Input: part model. Units: mm. Frame: model coordinates. Face numbers are marked on the shaded views. A direction names the side the tool comes from. Coordinates: 2 decimals unless noted, no trailing zeros. Loops run counter-clockwise (first coordinate to the right, second up) from the corner with the lowest first, then second, coordinate; pieces in that order, holes last. Notation, with made-up numbers: (-36.5, 69.5) - (-9.5, 69.5) arc R22 cw to (-9.5, 85.5) - close; hole circle Ø7 at (87, 70). An arc over 180 degrees is marked (long way). Use a Markdown table: item, result. Add a question column.
1. Draft query along X for the marked faces 1, 2 and 3. Return one class per face: released by +X, released by -X, zero draft, split by the parting line, or undercut.
2. Access query for the marked faces 4, 5 and 6. Directions: +Z, -Z, +X, -X, +Y, -Y. A direction counts if a zero-diameter tool reaches every point of the face in a straight line with its end or side. Return the directions, or none.
3. Ray query, L1, parallel to X at y = 1, z = -20; L2, parallel to X at y = 8.5, z = -13 (3 decimals); L3, parallel to Z at x = 38.5, y = -7 (3 decimals). Return the intervals inside material, ascending. Write a range as [from, to].
4. Section query C-C on z = 12. Return the cut outline in (x, y) (3 decimals), then the cut area to 3 significant figures.
5. Section query D-D on x = 21.5. Return the cut outline in (y, z) (3 decimals).
6. Contact query for flat-ended pins moving along their axis: P1, Ø4.5, axis at x = 52.125, z = 20.025, coming from the -Y side; P2, Ø3.5, axis at x = -45.5, z = 19, coming from the +Y side; P3, Ø1.5, axis at x = -12.5, z = -7.5, coming from the -Y side. Output: stop coordinate, or through.
7. Section query A-A on z = -7. Return the cut outline in (x, y) (3 decimals).
8. Section query B-B on y = 12. Return the cut outline in (x, z) (3 decimals), then the cut area to 3 significant figures.
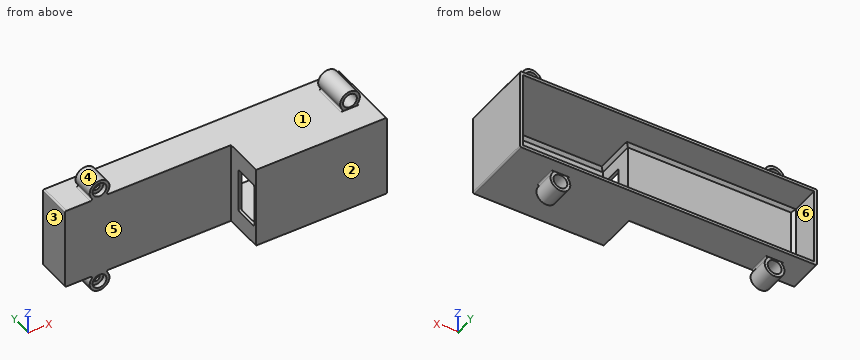
```python
from build123d import *

# Parameters (mm, degrees)
SKETCH1_W                      = 120.25
SKETCH1_H                      = 33.25
BOSS_EXTRUDE1_DEPTH            = 14
CUT_EXTRUDE1_REACH             = 67.133
CUT_EXTRUDE1_START             = 1.2
SKETCH1_3_W                    = 117.85
SKETCH1_3_H                    = 30.85
SKETCH2_W                      = 53
SKETCH2_H                      = 33.25
BOSS_EXTRUDE2_DEPTH            = 16
SKETCH2_3_W                    = 50.6
SKETCH2_3_H                    = 30.85
CUT_EXTRUDE2_DEPTH             = 14.8
CUT_EXTRUDE2_DIRECTION_2_REACH = 66.4
SKETCH3_W                      = 18
SKETCH3_H                      = 10
CUT_EXTRUDE4_DEPTH             = 8.325
SKETCH1_4_R                    = 4
BOSS_EXTRUDE3_DEPTH            = 9
BOSS_EXTRUDE4_START            = -5
SKETCH1_5_R                    = 4
BOSS_EXTRUDE4_DEPTH            = 5
CUT_EXTRUDE5_START             = 9
SKETCH1_6_R                    = 2.8
CUT_EXTRUDE5_DEPTH             = 6
CUT_EXTRUDE6_START             = 2
SKETCH1_7_R                    = 2.8
CUT_EXTRUDE6_DEPTH             = 7
CUT_EXTRUDE7_DEPTH             = 67.694949209
CUT_EXTRUDE7_DEPTH_BACK        = 67.694949209
SKETCH1_8_R                    = 1.3
CUT_EXTRUDE8_START             = 2
SKETCH1_9_R                    = 2.8
CUT_EXTRUDE8_DEPTH             = 2
FILLET1_R                      = 0.6
CHAMFER1_SIZE                  = 1.2


with BuildPart() as part:
    # Sketch1 → Boss-Extrude1 (new body)
    with BuildSketch(Plane(origin=(0, 0, 0), x_dir=(1, 0, 0), z_dir=(0, 1, 0))):
        Rectangle(SKETCH1_W, SKETCH1_H)
    extrude(amount=BOSS_EXTRUDE1_DEPTH)

    # Sketch1<3> → Cut-Extrude1 (cut, up to next)
    with BuildSketch(Plane(origin=(0, 0, 0), x_dir=(1, 0, 0), z_dir=(0, 1, 0)).offset(CUT_EXTRUDE1_START), mode=Mode.PRIVATE) as cut_extrude1_sk1:
        Rectangle(SKETCH1_3_W, SKETCH1_3_H)
    cut_extrude1_tool1 = extrude(cut_extrude1_sk1.sketch, amount=CUT_EXTRUDE1_REACH, mode=Mode.PRIVATE) & part.part
    add(cut_extrude1_tool1.solids().sort_by_distance((0, 1.2, 0))[0], mode=Mode.SUBTRACT)

    # Sketch2 → Boss-Extrude2 (add)
    with BuildSketch(Plane(origin=(0, 0, 0), x_dir=(1, 0, 0), z_dir=(0, 1, 0))):
        with Locations((33.625, 0)):
            Rectangle(SKETCH2_W, SKETCH2_H)
    extrude(amount=-BOSS_EXTRUDE2_DEPTH)

    # Sketch2<3> → Cut-Extrude2 (cut)
    with BuildSketch(Plane(origin=(0, 0, 0), x_dir=(1, 0, 0), z_dir=(0, 1, 0))):
        with Locations((33.625, 0)):
            Rectangle(SKETCH2_3_W, SKETCH2_3_H)
    extrude(amount=-CUT_EXTRUDE2_DEPTH, mode=Mode.SUBTRACT)

    # Sketch2<3> → Cut-Extrude2 direction 2 (cut, up to next)
    with BuildSketch(Plane(origin=(0, 0, 0), x_dir=(1, 0, 0), z_dir=(0, 1, 0)), mode=Mode.PRIVATE) as cut_extrude2_direction_2_sk1:
        with Locations((33.625, 0)):
            Rectangle(SKETCH2_3_W, SKETCH2_3_H)
    cut_extrude2_direction_2_tool1 = extrude(cut_extrude2_direction_2_sk1.sketch, amount=CUT_EXTRUDE2_DIRECTION_2_REACH, mode=Mode.PRIVATE) & part.part
    add(cut_extrude2_direction_2_tool1.solids().sort_by_distance((33.625, 0, 0))[0], mode=Mode.SUBTRACT)

    # Sketch3 → Cut-Extrude4 (cut)
    with BuildSketch(Plane(origin=(0, 0, 0), x_dir=(0, 0, -1), z_dir=(1, 0, 0))):
        with Locations((0, -9.8)):
            Rectangle(SKETCH3_W, SKETCH3_H)
    extrude(amount=CUT_EXTRUDE4_DEPTH, mode=Mode.SUBTRACT)

    # Sketch1<4> → Boss-Extrude3 (add)
    with BuildSketch(Plane(origin=(0, 0, 0), x_dir=(1, 0, 0), z_dir=(0, 1, 0))):
        with Locations((-46.125, -20.025)):
            Circle(SKETCH1_4_R)
        with Locations((52.125, -20.025)):
            Circle(SKETCH1_4_R)
        with Locations((-46.125, 20.025)):
            Circle(SKETCH1_4_R)
        with Locations((40.625, 20.025)):
            Circle(SKETCH1_4_R)
    extrude(amount=BOSS_EXTRUDE3_DEPTH)

    # Sketch1<5> → Boss-Extrude4 (add)
    with BuildSketch(Plane(origin=(0, 0, 0), x_dir=(1, 0, 0), z_dir=(0, 1, 0)).offset(BOSS_EXTRUDE4_START)):
        with Locations((52.125, -20.025)):
            Circle(SKETCH1_5_R)
    extrude(amount=BOSS_EXTRUDE4_DEPTH)

    # Sketch1<6> → Cut-Extrude5 (cut)
    with BuildSketch(Plane(origin=(0, 0, 0), x_dir=(1, 0, 0), z_dir=(0, 1, 0)).offset(CUT_EXTRUDE5_START)):
        with Locations(Location((-46.125, 20.025, 0), (0, 0, 270))):
            Circle(SKETCH1_6_R)
        with Locations(Location((-46.125, -20.025, 0), (0, 0, 270))):
            Circle(SKETCH1_6_R)
        with Locations(Location((52.125, -20.025, 0), (0, 0, 270))):
            Circle(SKETCH1_6_R)
        with Locations(Location((40.625, 20.025, 0), (0, 0, 270))):
            Circle(SKETCH1_6_R)
    extrude(amount=-CUT_EXTRUDE5_DEPTH, mode=Mode.SUBTRACT)

    # Sketch1<7> → Cut-Extrude6 (cut)
    with BuildSketch(Plane(origin=(0, 0, 0), x_dir=(1, 0, 0), z_dir=(0, 1, 0)).offset(CUT_EXTRUDE6_START)):
        with Locations(Location((52.125, -20.025, 0), (0, 0, 270))):
            Circle(SKETCH1_7_R)
    extrude(amount=-CUT_EXTRUDE6_DEPTH, mode=Mode.SUBTRACT)

    # Sketch1<8> → Cut-Extrude7 (cut, two sides: drawn at the far end of the back side and taken through both)
    with BuildSketch(Plane(origin=(0, 0, 0), x_dir=(1, 0, 0), z_dir=(0, 1, 0)).offset(-CUT_EXTRUDE7_DEPTH_BACK)):
        with Locations(Location((-46.125, 20.025, 0), (0, 0, 270))):
            Circle(SKETCH1_8_R)
        with Locations(Location((-46.125, -20.025, 0), (0, 0, 270))):
            Circle(SKETCH1_8_R)
        with Locations(Location((52.125, -20.025, 0), (0, 0, 270))):
            Circle(SKETCH1_8_R)
        with Locations(Location((40.625, 20.025, 0), (0, 0, 270))):
            Circle(SKETCH1_8_R)
    extrude(amount=CUT_EXTRUDE7_DEPTH + CUT_EXTRUDE7_DEPTH_BACK, mode=Mode.SUBTRACT)

    # Sketch1<9> → Cut-Extrude8 (cut)
    with BuildSketch(Plane(origin=(0, 0, 0), x_dir=(1, 0, 0), z_dir=(0, 1, 0)).offset(CUT_EXTRUDE8_START)):
        with Locations(Location((-46.125, 20.025, 0), (0, 0, 270))):
            Circle(SKETCH1_9_R)
        with Locations(Location((-46.125, -20.025, 0), (0, 0, 270))):
            Circle(SKETCH1_9_R)
        with Locations(Location((40.625, 20.025, 0), (0, 0, 270))):
            Circle(SKETCH1_9_R)
    extrude(amount=-CUT_EXTRUDE8_DEPTH, mode=Mode.SUBTRACT)

    # Fillet1
    fillet1_edges = [part.edges().sort_by_distance(p)[0] for p in [
        (7.725, -4.8, 9),
        (7.725, -14.8, 9),
        (7.725, -14.8, -9),
        (7.725, -4.8, -9),
        (54.232130751, 2, 16.625),
        (50.017869249, 2, 16.625),
        (60.125, -1, 16.625),
        (-48.232130751, 4.5, 16.625),
        (-44.017869249, 4.5, 16.625),
        (-60.125, 7, 16.625),
        (-60.125, 7, -16.625),
        (60.125, -1, -16.625),
        (42.732130751, 4.5, -16.625),
        (38.517869249, 4.5, -16.625),
        (-48.232130751, 4.5, -16.625),
        (-44.017869249, 4.5, -16.625),
    ]]
    fillet(fillet1_edges, radius=FILLET1_R)

    # Chamfer1
    chamfer1_edges = [part.edges().sort_by_distance(p)[0] for p in [
        (-58.925, 1.2, 0),
        (-25.3, 1.2, -15.425),
        (-25.3, 1.2, 15.425),
        (8.325, -6.8, -15.425),
        (8.325, -6.8, 15.425),
        (33.625, -14.8, 15.425),
        (58.925, -14.8, 0),
        (33.625, -14.8, -15.425),
    ]]
    chamfer(chamfer1_edges, length=CHAMFER1_SIZE)


solid = part.part
```
Resolved:
| question | item | result |
|---|---|---|
| 1 | face 1 | undercut |
| 1 | face 2 | zero draft |
| 1 | face 3 | released by -X |
| 2 | face 4 | +Y, -Y |
| 2 | face 5 | +Z, -Z, -X, -Y |
| 2 | face 6 | +Y |
| 3 | L1 | [-50.12, -48.92], [-43.33, -42.13], [36.63, 37.83], [43.42, 44.62] |
| 3 | L2 | [-60.125, -58.925], [58.925, 60.125] |
| 3 | L3 | [-16.625, -15.425], [15.425, 16.625] |
| 4 | outline | (-60.125, 0) - (7.125, 0) - (7.125, -16) - (60.125, -16) - (60.125, 14) - (58.925, 14) - (58.925, -13.6) - (57.725, -14.8) - (8.325, -14.8) - (8.325, 1.2) - (-57.725, 1.2) - (-58.925, 2.4) - (-58.925, 14) - (-60.125, 14) - close |
| 4 | area | 215 mm² |
| 5 | outline | (-16, -16.625) - (14, -16.625) - (14, -15.425) - (-13.6, -15.425) - (-14.8, -14.225) - (-14.8, 14.225) - (-13.6, 15.425) - (14, 15.425) - (14, 16.625) - (-16, 16.625) - close |
| 6 | P1 | y = 2 |
| 6 | P2 | y = 9 |
| 6 | P3 | y = 0 |
| 7 | outline | (-60.125, 0) - (7.125, 0) - (7.125, -4.8) - (8.325, -4.8) - (8.325, 1.2) - (-57.725, 1.2) - (-58.925, 2.4) - (-58.925, 14) - (-60.125, 14) - close; (7.125, -16) - (60.125, -16) - (60.125, 14) - (58.925, 14) - (58.925, -13.6) - (57.725, -14.8) - (7.125, -14.8) - close |
| 8 | outline | (-60.125, -16.025) arc R0.6 ccw to (-59.525, -16.625) - (59.525, -16.625) arc R0.6 ccw to (60.125, -16.025) - (60.125, 16.025) arc R0.6 ccw to (59.525, 16.625) - (-59.525, 16.625) arc R0.6 ccw to (-60.125, 16.025) - close; hole (-58.925, -15.425) - (58.925, -15.425) - (58.925, 15.425) - (-58.925, 15.425) - close |
| 8 | area | 362 mm² |
